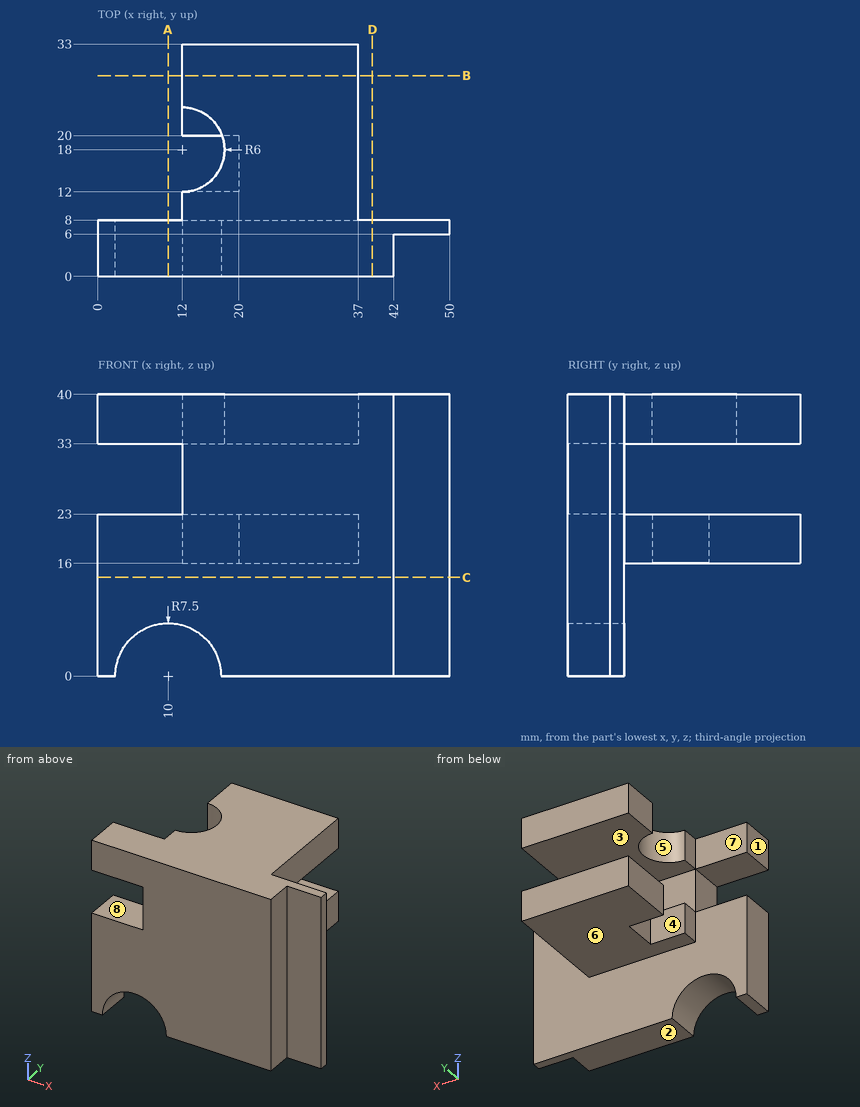
Geometry: see drawing. Coordinates: mm, zero at the bounding-box minimum. A direction names the side the tool comes from. Coordinates: 2 decimals unless noted, no trailing zeros. Loops run counter-clockwise (first coordinate to the right, second up) from the corner with the lowest first, then second, coordinate; pieces in that order, holes last. Notation, with made-up numbers: (57.25, -32.75) -> (99.25, -32.75) arc R5 ccw to (99.25, -23.75) -> close; hole circle Ø7 at (85.5, -30). An arc over 180 degrees is marked (long way). Use a Markdown table: item, result.
1) Cut plane D-D (x = 39). Return the cut outline in (y, z), then the cut area to 3 significant figures.
Results found:
| item | result |
|---|---|
| outline | (0, 0) -> (8, 0) -> (8, 40) -> (0, 40) -> close |
| area | 320 mm2 |
2) Contact query for flat-ended pins moving along their axis: pin 1 (1.5 mm diameter, centred on x = 37.5, y = 18, fed in from +Z); pin 2 (6.5 mm diameter, centred on x = 8.5, y = 5, fed in from -Z); pin 3 (2 mm diameter, centred on y = 28.5, z = 21, fed in from -X); pin 4 (3.5 mm diameter, centred on x = 7, z = 35, fed in from +Y). Output: stop coordinate, or through.
Results found:
| item | result |
|---|---|
| pin 1 | stops at z = 40 |
| pin 2 | stops at z = 5.8 |
| pin 3 | stops at x = 12 |
| pin 4 | stops at y = 8 |
3) Cut plane C-C (z = 14). Return the cut outline in (x, y).
Results found:
| item | result |
|---|---|
| outline | (0, 0) -> (42, 0) -> (42, 6) -> (50, 6) -> (50, 8) -> (0, 8) -> close |
4) Access query for the marked faces 4, 5, 6, 7 and 8. Directions: +Z, -Z, +X, -X, +Y, -Y. A direction counts if a zero-diameter tool reaches every point of the face in a straight line with its end or side. Return the directions, or none.
Results found:
| item | result |
|---|---|
| face 4 | -Z, -X |
| face 5 | +Z, -X |
| face 6 | -Z, +X, -X, +Y |
| face 7 | +Z, -Z, -X, +Y |
| face 8 | -X, +Y, -Y |
5) Material intervals for line 1 along Z through (x, y) = (26, 23.5); line 2 along X through (y, z) = (31, 19); line 3 along X through (y, z) = (19, 18.5), sorted ascending. Write a range as from..to.
Results found:
| item | result |
|---|---|
| line 1 | z = 16..23, 33..40 |
| line 2 | x = 12..37 |
| line 3 | x = 20..37 |
6) Pull-direction query (Z, two-part tool) for the marked faces 1, 2 and 3; classes: released by +Z, released by -Z, zero draft, split by the parting line, or undercut.
Results found:
| item | result |
|---|---|
| face 1 | zero draft |
| face 2 | released by -Z |
| face 3 | undercut |
7) Cut plane A-A (x = 10). Return the cut outline in (y, z).
Results found:
| item | result |
|---|---|
| outline | (0, 7.5) -> (8, 7.5) -> (8, 23) -> (0, 23) -> close; (0, 33) -> (8, 33) -> (8, 40) -> (0, 40) -> close |
8) Cut plane B-B (y = 28.5). Return the cut outline in (x, z).
Results found:
| item | result |
|---|---|
| outline | (12, 16) -> (37, 16) -> (37, 23) -> (12, 23) -> close; (12, 33) -> (37, 33) -> (37, 40) -> (12, 40) -> close |
